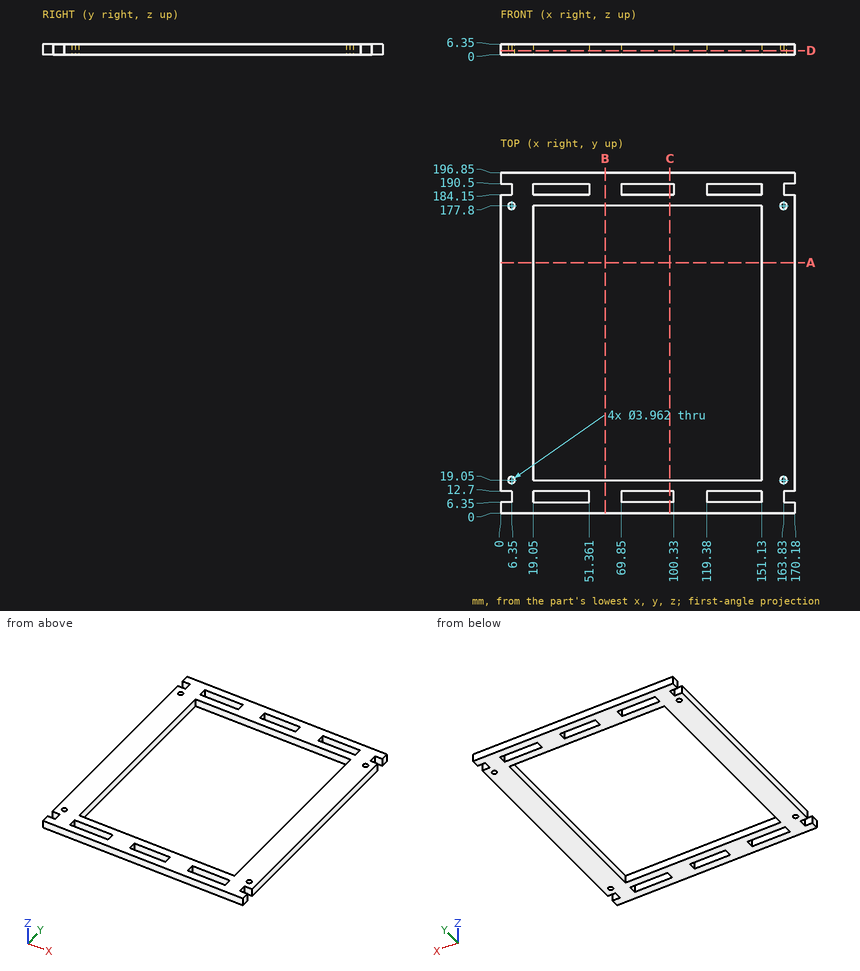
The figure shows three views and two pictorial views of one solid part (mm, origin at its lowest corner). Answer the questions. Round coordinates to 2 decimals unless told otherwise and drop trailing zeros. Order: outer loops, then holes, each group sorted by start corner. A loop starts at its lowest first (then second) coordinate and runs counter-clockwise, first axis right, second up.
Q1. Given pin 1 Ø1.9 at (x, z) = (84, 3) entering from -Y; pin 2 Ø1.9 at (y, z) = (188.5, 1.5) entering from +X; pin 3 Ø3 at (y, z) = (9, 3.5) entering from -X, each flat-ended and moving along its own axis, determine where each tip first touches the part or whether it passes through.
Solution:
pin 1: stops at y = 0
pin 2: stops at x = 163.83
pin 3: stops at x = 6.35
Q2. Find the intervals of material crossed by line 1 along Y through (x, z) = (124, 0.75); line 2 along Y through (x, z) = (61, 2.5); line 3 along X through (y, z) = (23.5, 4.5), in increasing order.
Solution:
line 1: y = 0 to 6.35, 12.7 to 19.05, 177.8 to 184.15, 190.5 to 196.85
line 2: y = 0 to 19.05, 177.8 to 196.85
line 3: x = 0 to 19.05, 151.13 to 170.18
Q3. A cutting plane is placed at D-D, the plane z = 2.5. Count the separate pieces of the cut face and the enclosed holes in it, then the cut area to 3 significant figures.
Solution:
separate pieces: 1
enclosed holes: 11
area: 11,100 mm2
Q4. A cutting plane is placed at A-A, the plane y = 145. Determine the outline of the cut face in (x, z), then the cut area to 3 significant figures.
Solution:
outline: (0, 0) - (19.05, 0) - (19.05, 6.35) - (0, 6.35) - close; (151.13, 0) - (170.18, 0) - (170.18, 6.35) - (151.13, 6.35) - close
area: 242 mm2
Q5. A cutting plane is placed at B-B, the plane x = 60.5. Determine the outline of the cut face in (y, z).
Solution:
outline: (0, 0) - (19.05, 0) - (19.05, 6.35) - (0, 6.35) - close; (177.8, 0) - (196.85, 0) - (196.85, 6.35) - (177.8, 6.35) - close
Q6. A cutting plane is placed at C-C, the plane x = 98. Determine the outline of the cut face in (y, z).
Solution:
outline: (0, 0) - (6.35, 0) - (6.35, 6.35) - (0, 6.35) - close; (12.7, 0) - (19.05, 0) - (19.05, 6.35) - (12.7, 6.35) - close; (177.8, 0) - (184.15, 0) - (184.15, 6.35) - (177.8, 6.35) - close; (190.5, 0) - (196.85, 0) - (196.85, 6.35) - (190.5, 6.35) - close
